Could you check a few things on this model? Use its own coordinates, in mm. Round coordinates to 2 decimals unless told otherwise and drop trailing zeros. Loops run counter-clockwise (first coordinate to the right, second up) from the corner with the lowest first, then second, coordinate; pieces in that order, holes last. Notation, with made-up numbers: (13.25, 19) -> (44.25, 19) arc R30 cw to (44.25, 54) -> close; hole circle Ø3 at (14, 42.5). An arc over 180 degrees is marked (long way). One line per item, written item: value.
Autodesk Inventor part; units mm, degrees
ref_plane "YZ Plane" through (0, 0, 0) normal (1, 0, 0) x (0, 1, 0)
ref_plane "XZ Plane" through (0, 0, 0) normal (0, 1, 0) x (-1, 0, 0)
ref_plane "XY Plane" through (0, 0, 0) normal (0, 0, 1) x (1, 0, 0)
sketch "Эскиз1" plane through (0, 0, 0) normal (0, 0, 1) x (1, 0, 0)
  line L0 (-119.1026, 5.3) -> (20.8974, 5.3)
  line L1 (20.8974, 5.3) -> (20.8974, 0)
  line L2 (20.8974, 0) -> (-119.1026, 0)
  line L3 (-119.1026, 0) -> (-119.1026, 5.3)
  point P0 (0, 0)
  point P1 (20.8974, 2.65)
  dimension "d0" = 5.3
  dimension "d1" = 140
extrude "Выдавливание1" add sketch "Эскиз1" along normal blind 1
sketch "Эскиз2" plane through (0, 0, 0) normal (0, 0, -1) x (-1, 0, 0)
  line L0 (-20.8974, 5.3) -> (119.1026, 5.3)
  line L1 (119.1026, 0) -> (-20.8974, 0)
  line L2 (119.1026, 5.3) -> (119.1026, 0)
  line L3 (-20.8974, 5.3) -> (119.1026, 5.3)
  line L4 (-20.8974, 0) -> (-20.8974, 5.3)
  line L5 (-20.8974, 0) -> (-20.8974, 5.3)
  line L6 (119.1026, 5.3) -> (119.1026, 0)
  line L7 (-20.8974, 5.3) -> (119.1026, 5.3)
  line L8 (119.1026, 5.3) -> (119.1026, 4.3)
  line L9 (119.1026, 4.3) -> (-20.8974, 4.3)
  line L10 (-20.8974, 4.3) -> (-20.8974, 5.3)
  line L11 (119.1026, 0) -> (-20.8974, 0)
  line L12 (-20.8974, 0) -> (-20.8974, 1)
  line L13 (-20.8974, 1) -> (119.1026, 1)
  line L14 (119.1026, 1) -> (119.1026, 0)
  point P0 (0, 0)
  dimension "d4" = 1
  dimension "d5" = 1
extrude "Выдавливание2" add sketch "Эскиз2" along normal blind 1.5 contours L0 L2 L9 L4 | L13 L2 L1 L4
properties part number "направляющая для стола"
(1) If we section it at C-C, the plane y = 3.3: Please give me the cut outline in (x, z).
Recorded:
outline: (-119.1, 0) -> (20.9, 0) -> (20.9, 1) -> (-119.1, 1) -> close
(2) If we section it at A-A, the plane z = -0.85: Please give me the cut outline in (x, y).
Recorded:
outline: (-119.1, 0) -> (20.9, 0) -> (20.9, 1) -> (-119.1, 1) -> close; (-119.1, 4.3) -> (20.9, 4.3) -> (20.9, 5.3) -> (-119.1, 5.3) -> close
(3) If we section it at B-B, the plane x = -54.5: Please give me the cut outline in (y, z).
Recorded:
outline: (0, -1.5) -> (1, -1.5) -> (1, 0) -> (4.3, 0) -> (4.3, -1.5) -> (5.3, -1.5) -> (5.3, 1) -> (0, 1) -> close
(4) If I drill on L1, parallel to Y at x = -89, z = -0.9; L2, parallel to Z at x = -98.5, y = 3.3, over which ranges is the centre line in solid material (lowest first)?
Recorded:
L1: 0 to 1, 4.3 to 5.3
L2: 0 to 1
(5) Thinking about a two-plate mould opening in Y: for faces 1 (the face through (-50, 5.3, 0)), 2 (the face through (-48, 0, 0)), 3 (the face through (-50, 3, 0)), which applies, released by +Y, released by -Y, zero draft, split by the parting line, or undercut?
Recorded:
face 1: released by +Y
face 2: released by -Y
face 3: undercut
